from build123d import *

# Parameters (mm, degrees)
SKETCH1_R                   = 38.1
OD_DON_T_CARE_DEPTH         = 25.4
SKETCH2_R                   = 4.7625
F_3_8_16_TAPPED_HOLES_DEPTH = 60.56828015
SKETCH4_R                   = 6.35
F_1_2_13_TAPPED_HOLE_DEPTH  = 60.56828015


with BuildPart() as part:
    # Sketch1 → OD Don't Care (new body)
    with BuildSketch(Plane.XY):
        Circle(SKETCH1_R)
    extrude(amount=OD_DON_T_CARE_DEPTH)

    # Sketch2 → 3/8"-16 Tapped Holes (cut, through all)
    with BuildSketch(Plane(origin=(0, 0, 0), x_dir=(-1, 0, 0), z_dir=(0, 0, -1))):
        with Locations((-25.4, 0)):
            Circle(SKETCH2_R)
        with Locations((25.4, 0)):
            Circle(SKETCH2_R)
    extrude(amount=-F_3_8_16_TAPPED_HOLES_DEPTH, mode=Mode.SUBTRACT)

    # Sketch4 → 1/2"-13 Tapped Hole (cut, through all)
    with BuildSketch(Plane(origin=(0, 0, 0), x_dir=(-1, 0, 0), z_dir=(0, 0, -1))):
        Circle(SKETCH4_R)
    extrude(amount=-F_1_2_13_TAPPED_HOLE_DEPTH, mode=Mode.SUBTRACT)


solid = part.part
Read the model definition and answer for the solid it produces. Units are mm, in the model's axes. Give positions to 0.01 mm unless a question says otherwise; leave off trailing zeros. Loops run counter-clockwise (first coordinate to the right, second up) from the corner with the lowest first, then second, coordinate; pieces in that order, holes last. Notation, with made-up numbers: M 32,63 L 39,63 A22 cw 39,77 Z; hole C 1,4 d8. An arc over 180 degrees is marked long. Write each question's results on one line, items separated by ' | '.
1. The mould has two halves that part along Y. Classify faces 1 (the face through (-30.235, -23.183, 12.522)), 2 (the face through (8, 1, 0)), 3 (the face through (21, -1.82, 12.52)): pulls with the +Y half, pulls with the -Y half, needs draft (parallel to the pull), parting line crosses it, or undercut.
Values:
face 1: parting line crosses it | face 2: needs draft | face 3: undercut
2. Section D-D on x = -25.4 is taken. Give the vertices of the cut face in (y, z).
Values:
outline: M -28.4,0 L -4.76,0 L -4.76,25.4 L -28.4,25.4 Z; M 4.76,0 L 28.4,0 L 28.4,25.4 L 4.76,25.4 Z
3. Section A-A on x = 0 is taken. Give the vertices of the cut face in (y, z), plus the area to 3 significant figures.
Values:
outline: M -38.1,0 L -6.35,0 L -6.35,25.4 L -38.1,25.4 Z; M 6.35,0 L 38.1,0 L 38.1,25.4 L 6.35,25.4 Z | area: 1,610 mm^2
4. Straight lines are drawn through the part: line 1 (Y direction, x = 0, z = 2.25); line 2 (Y direction, x = 1.5, z = 3.5); line 3 (Y direction, x = 19, z = 19). For each, find the intervals that lie inside material, in ascending order. Write a range as [from, to].
Values:
line 1: y = [-38.1, -6.35], [6.35, 38.1] | line 2: y = [-38.07, -6.17], [6.17, 38.07] | line 3: y = [-33.02, 33.02]
5. Section B-B on y = 0 is taken. Give the vertices of the cut face in (x, z).
Values:
outline: M -38.1,0 L -30.16,0 L -30.16,25.4 L -38.1,25.4 Z; M -20.64,0 L -6.35,0 L -6.35,25.4 L -20.64,25.4 Z; M 6.35,0 L 20.64,0 L 20.64,25.4 L 6.35,25.4 Z; M 30.16,0 L 38.1,0 L 38.1,25.4 L 30.16,25.4 Z
6. Section C-C on z = 19.5 is taken. State how many separate pieces and enclosed holes the cut face has, plus the area to 3 significant figures.
Values:
separate pieces: 1 | enclosed holes: 3 | area: 4,290 mm^2
7. Given pin 1 (1 mm diameter, centred on y = 6.5, z = 7, fed in from -X); pin 2 (10 mm diameter, centred on x = 4, z = 14.5, fed in from -Y); pin 3 (15 mm diameter, centred on x = 25.4, y = 0, fed in from -Z); pin 4 (10 mm diameter, centred on x = 3.5, z = 20, fed in from +Y), each flat-ended and moving along its own axis, determine where each tip first touches the part or whether it passes through.
Values:
pin 1: stops at x = -37.62 | pin 2: stops at y = -38.1 | pin 3: stops at z = 0 | pin 4: stops at y = 38.1
